```python
from build123d import *

# Parameters (mm, degrees)
F1_DEPTH       = 15
F2_DEPTH       = 2
F4_D           = 3
F4_DEPTH       = 100
F4_CBORE_D     = 10
F4_CBORE_DEPTH = 0.2
F4_TIP         = 0.9012909285
F5_T1_DEPTH    = 15
F5_T6_DEPTH    = 13
F5_S7_R        = 5
F5_T8_DEPTH    = 9
F5_T9_DEPTH    = 40.7168298797
F5_T11_DEPTH   = 27.7168298797
F6_R           = 1


# Not quite as in the source:
# - a fillet or chamfer that OpenCascade refuses, or shapes differently, is made with other operations: its cross-section is extruded or revolved along the edge and cut away or added


with BuildPart() as f1:
    # F0 (on Right) → F1 (new body)
    with BuildSketch(Plane.YZ):
        Polygon((-35, 9), (-35, 0), (0, 0), (0, 7.5), (0, 15), (6.5, 15), (13, 15), (13, 17), (-2, 17), (-2, 2), (-33, 2), (-33, 9), align=None)
    extrude(amount=F1_DEPTH)

    # F0 (on Right) → F2 (join)
    with BuildSketch(Plane.YZ):
        Polygon((0, 15), (0, 7.5), (6.5, 15), align=None)
    extrude(amount=F2_DEPTH)

    # F4
    with Locations(Plane(origin=(0, 0, 15), x_dir=(1, 0, 0), z_dir=(0, 0, -1))):
        with Locations((7.5, -5.5)):
            CounterBoreHole(F4_D / 2, F4_CBORE_D / 2, F4_CBORE_DEPTH, depth=F4_DEPTH)
            with Locations((0, 0, -(F4_DEPTH + F4_TIP / 2))):  # 118° drill point
                Cone(0, F4_D / 2, F4_TIP, mode=Mode.SUBTRACT)

    # F5: chamfer of 5 on 7 edges, made by hand

    # F5_s2 → F5_t1 (join)
    with BuildSketch(Plane.YZ):
        Polygon((-2, 7), (-7, 2), (-2, 2), align=None)
        Polygon((-33, 7), (-28, 2), (-33, 2), align=None)
    extrude(amount=F5_T1_DEPTH)


with BuildPart() as f5_tool4:
    # F5_s5 → F5_t6 (new body)
    with BuildSketch(Plane.YZ.offset(2)):
        Polygon((0, 10), (5, 15), (0, 15), align=None)
    extrude(amount=F5_T6_DEPTH)

    # F5_s7 → F5_t8 (cut, symmetric)
    with BuildSketch(Plane.XY.offset(12.5)):
        with Locations((7.5, 5.5)):
            Circle(F5_S7_R)
    extrude(amount=F5_T8_DEPTH, both=True, mode=Mode.SUBTRACT)


with BuildPart() as f1_1:
    add(f1.part)

    # F5_t3: union F5_tool4
    add(f5_tool4.part)

    # F5_s10 → F5_t9 (cut)
    with BuildSketch(Plane.YZ.offset(-12.8584149398)):
        Polygon((-35, 5), (-30, 0), (-35, 0), align=None)
        Polygon((-5, 0), (0, 5), (0, 0), align=None)
    extrude(amount=F5_T9_DEPTH, mode=Mode.SUBTRACT)

    # F5_s12 → F5_t11 (cut)
    with BuildSketch(Plane.XY.offset(2.1415850602)):
        Polygon((15, 8), (10, 13), (15, 13), align=None)
        Polygon((0, 8), (5, 13), (0, 13), align=None)
    extrude(amount=F5_T11_DEPTH, mode=Mode.SUBTRACT)

    # F6
    f6_edges = [f1_1.edges().sort_by_distance(p)[0] for p in [
        (7.5, -35, 9),
        (7.5, 0, 5),
        (7.5, -5, 0),
        (7.5, -30, 0),
        (7.5, -35, 5),
        (7.5, -33, 7),
        (7.5, -28, 2),
        (7.5, -7, 2),
        (7.5, -2, 7),
    ]]
    fillet(f6_edges, radius=F6_R)


solid = f1_1.part
```
Geometry: final body of the model. Coordinates: model frame, mm. A direction names the side the tool comes from. Round coordinates to 2 decimals unless told otherwise and drop trailing zeros. Order: outer loops, then holes, each group sorted by start corner. A loop starts at its lowest first (then second) coordinate and runs counter-clockwise, first axis right, second up. Notation, with made-up numbers: (5, 32) -> (51, 32) arc R21 ccw to (51, 40) -> close; hole circle Ø8 at (0.5, 40.25). An arc over 180 degrees is marked (long way). Use one line per item in the form item = value.
(1) Section D-D on x = 4. Return loops of the section in (y, z), and give its area (3 significant figures).
Results list:
outline = (-35, 5.41) arc R1 ccw to (-34.71, 4.71) -> (-30.29, 0.29) arc R1 ccw to (-29.59, 0) -> (-5.41, 0) arc R1 ccw to (-4.71, 0.29) -> (-0.29, 4.71) arc R1 ccw to (0, 5.41) -> (0, 10) -> (1.93, 11.93) -> (1.93, 15.2) -> (9.07, 15.2) -> (9.07, 15) -> (12, 15) -> (12, 17) -> (-2, 17) -> (-2, 7.41) arc R1 cw to (-2.29, 6.71) -> (-6.71, 2.29) arc R1 cw to (-7.41, 2) -> (-27.59, 2) arc R1 cw to (-28.29, 2.29) -> (-32.71, 6.71) arc R1 cw to (-33, 7.41) -> (-33, 9) -> (-34, 9) arc R1 ccw to (-35, 8) -> close
area = 144 mm^2
(2) Ray query, probe 1 along Y at (x, z) = (7.5, 15.75); probe 2 along Z at (x, y) = (6.25, 0.5); probe 3 along Y at (x, z) = (12.25, 10.5). Return the intervals inside material, ascending. Write a range as [from, to].
Results list:
probe_1 = [-2, 4], [7, 13]
probe_2 = [10.5, 17]
probe_3 = [-2, 0.5]
(3) Access query for faces 4 (the face through (9, 4, 15.2)), 5 (the face through (2, 3, 12)), 6 (the face through (7, -33, 8)). Directions: +Z, -Z, +X, -X, +Y, -Y. A direction counts if a zero-diameter tool reaches every point of the face in a straight line with its end or side. Return the directions, or none.
Results list:
face_4 = -Z
face_5 = -Z, +X, +Y
face_6 = +Z, +X, -X
(4) Section B-B on y = 5.5. Return loops of the section in (x, z).
Results list:
outline = (0, 13.85) -> (2, 13.85) -> (2, 15) -> (2.5, 15) -> (2.5, 15.2) -> (6, 15.2) -> (6, 17) -> (0, 17) -> close; (9, 15.2) -> (12.5, 15.2) -> (12.5, 15) -> (15, 15) -> (15, 17) -> (9, 17) -> close
(5) Section C-C on z = 14.5. Return loops of the section in (x, y), and give its area (3 significant figures).
Results list:
outline = (0, -2) -> (15, -2) -> (15, 4.5) -> (12.4, 4.5) arc R5 cw to (2.6, 4.5) -> (2, 4.5) -> (2, 6.07) -> (0, 6.07) -> close
area = 71.3 mm^2
(6) Draft query along X for faces 1 (the face through (9, 5.43, 16.11)), 2 (the face through (2, 10, 16)), 3 (the face through (7, -2, 12)). Return one class per face: pulls with the +X half, pulls with the -X half, needs draft (parallel to the pull), parting line crosses it, or undercut.
Results list:
face_1 = undercut
face_2 = pulls with the -X half
face_3 = needs draft
(7) First-contact query: pin 1 Ø1.7 at (x, z) = (4, 8.5) entering from +Y; pin 2 Ø4 at (x, y) = (9, 7.5) entering from -Z; pin 3 Ø7.5 at (x, y) = (9, -20) entering from +Z; pin 4 Ø4 at (y, z) = (-16, 5.5) entering from -X (1 decimal). Flat tips, straight axial feed; report the tip coordinate or a pass-through.
Results list:
pin_1 = 0
pin_2 = 15.2
pin_3 = 2
pin_4 = through
